Work out the finished part from the listing and answer in its coordinate system (mm). Face numbers are marked on the shaded views. A direction names the side the tool comes from. Round coordinates to 2 decimals unless told otherwise and drop trailing zeros. Order: outer loops, then holes, each group sorted by start corner. A loop starts at its lowest first (then second) coordinate and runs counter-clockwise, first axis right, second up. Notation, with made-up numbers: (-1, -33.5) - (46, -33.5) arc R35 ccw to (46, -1.5) - close; hole circle Ø4 at (74, 89). An arc over 180 degrees is marked (long way). Answer in a Markdown table with one row per item.
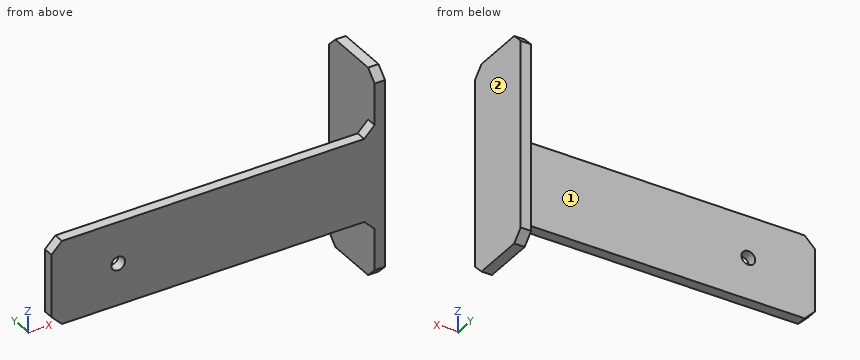
from build123d import *

# Parameters (mm, degrees)
SKETCH1_W           = 160
SKETCH1_H           = 40
SKETCH1_R           = 3.302
BOSS_EXTRUDE1_DEPTH = 5
SKETCH2_W           = 5
SKETCH2_H           = 100
BOSS_EXTRUDE2_DEPTH = 35
CHAMFER1_SIZE       = 5


with BuildPart() as part:
    # Sketch1 → Boss-Extrude1 (new body)
    with BuildSketch(Plane(origin=(0, 0, 0), x_dir=(1, 0, 0), z_dir=(0, 1, 0))):
        with Locations((80, 20)):
            Rectangle(SKETCH1_W, SKETCH1_H)
        with Locations(Location((32, 20, 0), (0, 0, 270))):
            Circle(SKETCH1_R, mode=Mode.SUBTRACT)
    extrude(amount=BOSS_EXTRUDE1_DEPTH)

    # Sketch2 → Boss-Extrude2 (add)
    with BuildSketch(Plane.XZ):
        with Locations((157.5, -20)):
            Rectangle(SKETCH2_W, SKETCH2_H)
    extrude(amount=-BOSS_EXTRUDE2_DEPTH)

    # Chamfer1
    chamfer1_edges = [part.edges().sort_by_distance(p)[0] for p in [
        (155, 2.5, -40),
        (157.5, 0, 30),
        (157.5, 0, -70),
        (155, 2.5, 0),
        (157.5, 35, 30),
        (157.5, 35, -70),
        (0, 2.5, -40),
        (0, 2.5, 0),
    ]]
    chamfer(chamfer1_edges, length=CHAMFER1_SIZE)


solid = part.part
1) Find section D-D, the plane y = 24. Give the vertices of the cut face in (x, z), then the cut area to 3 significant figures.
Filled in:
| item | result |
|---|---|
| outline | (155, -70) - (160, -70) - (160, 30) - (155, 30) - close |
| area | 500 mm^2 |
2) Which of the six approach directions +Z, -Z, +X, -X, +Y, -Y give full straight-line access (tool end or side, diameter ignored) to the marked faces 1 and 2?
Filled in:
| item | result |
|---|---|
| face 1 | +Z, -Z, -X, +Y |
| face 2 | +Z, -Z, +X, +Y, -Y |
3) Find the intervals of material crossed by probe 1 along X at (y, z) = (1.1, -20); probe 2 along Y at (x, z) = (64, -25); probe 3 along X at (y, z) = (19.5, 11), in increasing order. Write a range as from..to.
Filled in:
| item | result |
|---|---|
| probe 1 | x = 0..28.7, 35.3..160 |
| probe 2 | y = 0..5 |
| probe 3 | x = 155..160 |
4) Find section C-C, the plane z = 16.5. Give the vertices of the cut face in (x, y), then the cut area to 3 significant figures.
Filled in:
| item | result |
|---|---|
| outline | (155, 0) - (160, 0) - (160, 35) - (155, 35) - close |
| area | 175 mm^2 |
5) Find section A-A, the plane x = 32. Give the vertices of the cut face in (y, z).
Filled in:
| item | result |
|---|---|
| outline | (0, -40) - (5, -40) - (5, -23.3) - (0, -23.3) - close; (0, -16.7) - (5, -16.7) - (5, 0) - (0, 0) - close |
6) Find section B-B, the plane z = -20. Give the vertices of the cut face in (x, y), then the cut area to 3 significant figures.
Filled in:
| item | result |
|---|---|
| outline | (0, 0) - (28.7, 0) - (28.7, 5) - (0, 5) - close; (35.3, 0) - (160, 0) - (160, 35) - (155, 35) - (155, 5) - (35.3, 5) - close |
| area | 917 mm^2 |
7) Each of these flat-tipped pins is pushed along its axis until it touches: pin 1 (8 mm diameter, centred on y = 23.5, z = -16.5, fed in from -X); pin 2 (2.5 mm diameter, centred on x = 46, y = 3, fed in from +Z); pin 3 (1.5 mm diameter, centred on x = 65, y = 2.5, fed in from -Z); pin 4 (5.5 mm diameter, centred on x = 32, z = -20, fed in from +Y). Where does it stop, or does it pass through?
Filled in:
| item | result |
|---|---|
| pin 1 | stops at x = 155 |
| pin 2 | stops at z = 0 |
| pin 3 | stops at z = -40 |
| pin 4 | passes through |
